from build123d import *

# Parameters (mm, degrees)
SKETCH1_W           = 40
SKETCH1_H           = 40
BOSS_EXTRUDE1_DEPTH = 6
SKETCH2_W           = 40
SKETCH2_H           = 40
SKETCH2_R           = 4.5
BOSS_EXTRUDE2_DEPTH = 3
SKETCH3_R           = 2.5
CUT_EXTRUDE1_DEPTH  = 24
SKETCH4_R           = 7.5
SKETCH4_R_2         = 4.5
BOSS_EXTRUDE3_DEPTH = 7
FILLET1_R           = 3
CHAMFER1_SIZE       = 5


with BuildPart() as part:
    # Sketch1 → Boss-Extrude1 (new body)
    with BuildSketch(Plane(origin=(0, 0, 0), x_dir=(1, 0, 0), z_dir=(0, 1, 0))):
        Rectangle(SKETCH1_W, SKETCH1_H)
        Polygon((7.505553499, 0), (3.75277675, 6.5), (-3.75277675, 6.5), (-7.505553499, 0), (-3.75277675, -6.5), (3.75277675, -6.5), align=None, mode=Mode.SUBTRACT)
    extrude(amount=BOSS_EXTRUDE1_DEPTH)

    # Sketch2 → Boss-Extrude2 (add)
    with BuildSketch(Plane(origin=(0, 6, 0), x_dir=(1, 0, 0), z_dir=(0, 1, 0))):
        Rectangle(SKETCH2_W, SKETCH2_H)
        with Locations(Location((0, 0, 0), (0, 0, 270))):
            Circle(SKETCH2_R, mode=Mode.SUBTRACT)
    extrude(amount=BOSS_EXTRUDE2_DEPTH)

    # Sketch3 → Cut-Extrude1 (cut)
    with BuildSketch(Plane(origin=(0, 9, 0), x_dir=(1, 0, 0), z_dir=(0, 1, 0))):
        with Locations(Location((-11.514718626, 11.514718626, 0), (0, 0, 270))):
            Circle(SKETCH3_R)
        with Locations(Location((11.514718626, 11.514718626, 0), (0, 0, 270))):
            Circle(SKETCH3_R)
        with Locations(Location((11.514718626, -11.514718626, 0), (0, 0, 270))):
            Circle(SKETCH3_R)
        with Locations(Location((-11.514718626, -11.514718626, 0), (0, 0, 270))):
            Circle(SKETCH3_R)
    extrude(amount=-CUT_EXTRUDE1_DEPTH, mode=Mode.SUBTRACT)

    # Sketch4 → Boss-Extrude3 (add)
    with BuildSketch(Plane(origin=(0, 9, 0), x_dir=(1, 0, 0), z_dir=(0, 1, 0))):
        with Locations(Location((0, 0, 0), (0, 0, 90))):
            Circle(SKETCH4_R)
        with Locations(Location((0, 0, 0), (0, 0, 270))):
            Circle(SKETCH4_R_2, mode=Mode.SUBTRACT)
    extrude(amount=BOSS_EXTRUDE3_DEPTH)

    # Fillet1
    fillet1_edges = [part.edges().sort_by_distance(p)[0] for p in [
        (0, 9, 7.5),
    ]]
    fillet(fillet1_edges, radius=FILLET1_R)

    # Chamfer1
    chamfer1_edges = [part.edges().sort_by_distance(p)[0] for p in [
        (20, 4.5, 20),
        (-20, 4.5, 20),
        (-20, 4.5, -20),
        (20, 4.5, -20),
    ]]
    chamfer(chamfer1_edges, length=CHAMFER1_SIZE)


solid = part.part
The model under review builds one solid part; all positions refer to its coordinate system, in mm. A direction names the side the tool comes from. Coordinates: 2 decimals unless noted, no trailing zeros. Write each loop counter-clockwise with the first axis right and the second up, starting at its lowest first coordinate (ties: lowest second). Pieces come first, ordered by that corner, then holes. Notation, with made-up numbers: M -14,-36.5 L -6,-36.5 A27 ccw -6,-13.5 Z; hole C -4.75,-28.5 d6. An arc over 180 degrees is marked long. Put each result on its own line as item: value.
1) Add section D-D on x = -12. Give the boundary of the cut face in (y, z), then the cut area to 3 significant figures.
Computed:
outline: M 0,-20 L 9,-20 L 9,-13.97 L 0,-13.97 Z; M 0,-9.06 L 9,-9.06 L 9,9.06 L 0,9.06 Z; M 0,13.97 L 9,13.97 L 9,20 L 0,20 Z
area: 272 mm2
2) Add section B-B on z = -12. Give the boundary of the cut face in (x, y), then the cut area to 3 significant figures.
Computed:
outline: M -20,0 L -13.97,0 L -13.97,9 L -20,9 Z; M -9.06,0 L 9.06,0 L 9.06,9 L -9.06,9 Z; M 13.97,0 L 20,0 L 20,9 L 13.97,9 Z
area: 272 mm2
3) Draft analysis for pull direction X (two halves, no side actions). For faces 4 (the flat face through (-17, 5, -18)), 5 (the cylindrical face through (11.625, 4.563, -14.012)), 6 (the flat face through (-5.66, 2.96, 3.2)), 7 (the flat face through (20, 4, 0)), state which applies: released by +X, released by -X, zero draft, split by the parting line, or undercut.
Computed:
face 4: released by -X
face 5: undercut
face 6: undercut
face 7: released by +X
4) Clearance check with flat-ended pins moving along their axes: pin 1 Ø10.5 at (x, z) = (1.5, 2.5) entering from -Y; pin 2 Ø6 at (x, z) = (1, 2) entering from -Y; pin 3 Ø3 at (x, y) = (-7.5, 11) entering from -Z. State where each tip first meets the part, or that it passes through.
Computed:
pin 1: stops at y = 0
pin 2: stops at y = 6
pin 3: stops at z = -5.29
5) Wall thickness on probe 1 along X at (y, z) = (12.75, 0); probe 2 along X at (y, z) = (2.5, -9.5); probe 3 along Y at (x, z) = (11.5, 1.5): over which ranges is each line inside the solid? List them lowest first. Write a range as [from, to].
Computed:
probe 1: x = [-7.5, -4.5], [4.5, 7.5]
probe 2: x = [-20, -12.99], [-10.03, 10.03], [12.99, 20]
probe 3: y = [0, 9]
6) Add section C-C on y = 2.5. Give the boundary of the cut face in (x, z).
Computed:
outline: M -20,-15 L -15,-20 L 15,-20 L 20,-15 L 20,15 L 15,20 L -15,20 L -20,15 Z; hole C -11.51,-11.51 d5; hole C -11.51,11.51 d5; hole M -7.51,0 L -3.75,-6.5 L 3.75,-6.5 L 7.51,0 L 3.75,6.5 L -3.75,6.5 Z; hole C 11.51,-11.51 d5; hole C 11.51,11.51 d5
7) Add section A-A on x = 0. Give the boundary of the cut face in (y, z).
Computed:
outline: M 0,-20 L 9,-20 L 9,-10.5 A3 cw 12,-7.5 L 16,-7.5 L 16,-4.5 L 6,-4.5 L 6,-6.5 L 0,-6.5 Z; M 0,6.5 L 6,6.5 L 6,4.5 L 16,4.5 L 16,7.5 L 12,7.5 A3 cw 9,10.5 L 9,20 L 0,20 Z
8) For faces 1 (the flat face through (9, 9, 9)), 2 (the cylindrical face through (11.625, 4.563, 9.017)), 3 (the flat face through (0, 3, -6.5)), list the 3-axis set-ups (+Z, -Z, +X, -X, +Y, -Y) from which the entire face can be reached by the end or side of a thin tool; tool diameter is ignored.
Computed:
face 1: +Y
face 2: +Y, -Y
face 3: -Y
